The listing builds one solid part. Answer for the finished solid, in the listing's coordinates (mm). A direction names the side the tool comes from. Give positions to 0.01 mm unless a question says otherwise; leave off trailing zeros. Order: outer loops, then holes, each group sorted by start corner. A loop starts at its lowest first (then second) coordinate and runs counter-clockwise, first axis right, second up. Notation, with made-up numbers: (53.5, 17.25) - (84.5, 17.25) arc R28 ccw to (84.5, 45.25) - close; hole circle Ø7 at (25, 16.25). An arc over 180 degrees is marked (long way). Answer in a Markdown table with one row per item.
from build123d import *

# Parameters (mm, degrees)
F1_DEPTH = 71.12
F3_DEPTH = 101.6
F5_DEPTH = 78.614


with BuildPart() as f1:
    # F0 (on Top) → F1 (new body)
    with BuildSketch(Plane.XY):
        with BuildLine():
            Line((-92.075, 0), (0, 0))
            Line((0, 0), (92.075, 0))
            Line((92.075, 0), (92.075, 4.191))
            ThreePointArc((92.075, 4.191), (87.438941, 16.646554), (75.78725, 23.039673))
            ThreePointArc((75.78725, 23.039673), (71.903353, 25.170713), (70.358, 29.322564))
            Line((70.358, 29.322564), (70.358, 41.662933))
            ThreePointArc((70.358, 41.662933), (70.60499, 42.890688), (71.307533, 43.927424))
            ThreePointArc((71.307533, 43.927424), (79.625637, 56.202377), (82.55, 70.739))
            Line((82.55, 70.739), (82.55, 74.549))
            Line((82.55, 74.549), (78.0415, 74.549))
            Line((78.0415, 74.549), (78.0415, 77.089))
            Line((78.0415, 77.089), (81.2165, 77.089))
            Line((81.2165, 77.089), (81.2165, 78.613))
            Line((81.2165, 78.613), (78.0415, 78.613))
            Line((78.0415, 78.613), (75.5015, 78.613))
            Line((75.5015, 78.613), (75.5015, 74.549))
            Line((75.5015, 74.549), (70.993, 74.549))
            Line((70.993, 74.549), (70.993, 70.739))
            Line((70.993, 70.739), (73.867173, 70.739))
            ThreePointArc((73.867173, 70.739), (76.23161, 69.682976), (77.023196, 67.217384))
            ThreePointArc((77.023196, 67.217384), (74.034342, 56.769573), (67.745761, 47.907082))
            ThreePointArc((67.745761, 47.907082), (65.731431, 44.897155), (65.024, 41.345152))
            Line((65.024, 41.345152), (65.024, 29.591))
            ThreePointArc((65.024, 29.591), (63.164128, 25.100872), (58.674, 23.241))
            Line((58.674, 23.241), (0, 23.241))
            Line((0, 23.241), (-58.674, 23.241))
            ThreePointArc((-58.674, 23.241), (-63.164128, 25.100872), (-65.024, 29.591))
            Line((-65.024, 29.591), (-65.024, 41.345152))
            ThreePointArc((-65.024, 41.345152), (-65.731431, 44.897155), (-67.745761, 47.907082))
            ThreePointArc((-67.745761, 47.907082), (-74.034342, 56.769573), (-77.023196, 67.217384))
            ThreePointArc((-77.023196, 67.217384), (-76.23161, 69.682976), (-73.867173, 70.739))
            Line((-73.867173, 70.739), (-70.993, 70.739))
            Line((-70.993, 70.739), (-70.993, 74.549))
            Line((-70.993, 74.549), (-75.5015, 74.549))
            Line((-75.5015, 74.549), (-75.5015, 78.613))
            Line((-75.5015, 78.613), (-81.2165, 78.613))
            Line((-81.2165, 78.613), (-81.2165, 77.089))
            Line((-81.2165, 77.089), (-78.0415, 77.089))
            Line((-78.0415, 77.089), (-78.0415, 74.549))
            Line((-78.0415, 74.549), (-82.55, 74.549))
            Line((-82.55, 74.549), (-82.55, 70.739))
            ThreePointArc((-82.55, 70.739), (-79.625637, 56.202377), (-71.307533, 43.927424))
            ThreePointArc((-71.307533, 43.927424), (-70.60499, 42.890688), (-70.358, 41.662933))
            Line((-70.358, 41.662933), (-70.358, 29.322564))
            ThreePointArc((-70.358, 29.322564), (-71.903353, 25.170713), (-75.78725, 23.039673))
            ThreePointArc((-75.78725, 23.039673), (-87.438941, 16.646554), (-92.075, 4.191))
            Line((-92.075, 4.191), (-92.075, 0))
        make_face()
    extrude(amount=F1_DEPTH)

    # F2 (on Right) → F3 (intersect, symmetric)
    with BuildSketch(Plane.YZ):
        with BuildLine():
            Line((0.047138, 2.79405), (0, 0))
            Line((0, 0), (23.240988, 0.02372))
            ThreePointArc((23.240988, 0.02372), (55.450197, 9.625805), (75.869463, 36.322))
            Line((75.869463, 36.322), (78.613, 36.322))
            Line((78.613, 36.322), (78.613, 71.12407))
            Line((78.613, 71.12407), (74.6252, 71.12))
            ThreePointArc((74.6252, 71.12), (59.575116, 34.785884), (23.241, 19.7358))
            Line((23.241, 19.7358), (19.859128, 19.7358))
            Line((19.859128, 19.7358), (19.859128, 2.81427))
            Line((19.859128, 2.81427), (0.047138, 2.79405))
        make_face()
    extrude(amount=F3_DEPTH, both=True, mode=Mode.INTERSECT)

    # F4 (on Front) → F5 (cut, through all)
    with BuildSketch(Plane.XZ):
        with BuildLine():
            Line((-85.773818, 62.544154), (-82.55, 62.544154))
            ThreePointArc((-82.55, 62.544154), (-76.7715, 68.322654), (-70.993, 62.544154))
            Line((-70.993, 62.544154), (-67.021526, 62.544154))
            Line((-67.021526, 62.544154), (-67.021526, 73.423296))
            Line((-67.021526, 73.423296), (-85.773818, 73.423296))
            Line((-85.773818, 73.423296), (-85.773818, 62.544154))
        make_face()
        with BuildLine():
            ThreePointArc((70.993, 62.544154), (76.7715, 68.322654), (82.55, 62.544154))
            Line((82.55, 62.544154), (85.773818, 62.544154))
            Line((85.773818, 62.544154), (85.773818, 73.423296))
            Line((85.773818, 73.423296), (67.021526, 73.423296))
            Line((67.021526, 73.423296), (67.021526, 62.544154))
            Line((67.021526, 62.544154), (70.993, 62.544154))
        make_face()
    extrude(amount=-F5_DEPTH, mode=Mode.SUBTRACT)


solid = f1.part
Item 1: Find section A-A on y = 53. Write down the section's boundary in (x, z).
Answer block:
| item | result |
|---|---|
| outline | (-78.1, 8.03) - (-71.9, 8.03) - (-71.9, 29.23) - (-78.1, 29.23) - close; (71.9, 8.03) - (78.1, 8.03) - (78.1, 29.23) - (71.9, 29.23) - close |
Item 2: Determine the mould class of faces 6 (the face through (79.544, 56.01, 21.881)), 7 (the face through (-65.024, 35, 11)), 8 (the face through (1, 19.859, 11)) for opening direction Y: pulls with the +Y half, pulls with the -Y half, needs draft (parallel to the pull), parting line crosses it, or undercut.
Answer block:
| item | result |
|---|---|
| face 6 | undercut |
| face 7 | needs draft |
| face 8 | pulls with the -Y half |
Item 3: Consider line 1 (X direction, y = 36.5, z = 19.5); line 2 (Y direction, x = 19, z = 16); line 3 (Z direction, x = -57, y = 18.5). Determine where each line is inside the solid, lowest interval first.
Answer block:
| item | result |
|---|---|
| line 1 | -70.36 to -65.02, 65.02 to 70.36 |
| line 2 | 19.86 to 23.24 |
| line 3 | 0.02 to 2.81 |
Item 4: Find section D-D on y = 26.5. Write down the section's boundary in (x, z), then the cut area to 3 significant figures.
Answer block:
| item | result |
|---|---|
| outline | (-71.02, 0.04) - (-64.22, 0.04) - (-64.22, 19.84) - (-71.02, 19.84) - close; (64.22, 0.04) - (71.02, 0.04) - (71.02, 19.84) - (64.22, 19.84) - close |
| area | 269 mm² |
Item 5: Which of the six approach directions +Z, -Z, +X, -X, +Y, -Y give full straight-line access (tool end or side, diameter ignored) to faces 1 (the face through (-70.358, 36, 12)), 2 (the face through (80, 74.549, 50)), 3 (the face through (-73, 74.549, 50)), 4 (the face through (74.1, 56.91, 24.63)), 5 (the face through (1, 22, 19.736))?
Answer block:
| item | result |
|---|---|
| face 1 | +Z, -Z, -X |
| face 2 | +Z, -Z, +X |
| face 3 | +Z, -Z, +Y |
| face 4 | +Z, -Z |
| face 5 | +Z, +X, -X, -Y |
Item 6: Each of these flat-tipped pins is pushed along its axis until it touches: P1, Ø1.9, axis at y = 73, z = 37.5, coming from the -X side; P2, Ø1.6, axis at x = -79, z = 50.5, coming from the -Y side; P3, Ø18.5, axis at x = -6.5, z = 12, coming from the -Y side. Where does it stop, or does it pass through?
Answer block:
| item | result |
|---|---|
| P1 | x = -82.55 |
| P2 | y = 69.95 |
| P3 | y = 0.05 |
